```python
from build123d import *

# Parameters (mm, degrees)
EXTRUDE_1_DEPTH     = 6
SKETCH_2_W          = 1
SKETCH_2_H          = 3.5
CUT_EXTRUDE_1_DEPTH = 30.086079144
SKETCH_3_W          = 1
SKETCH_3_H          = 3.5
CUT_EXTRUDE_2_DEPTH = 6


with BuildPart() as part:
    # 草图1 → 凸台-拉伸1 (new body)
    with BuildSketch(Plane(origin=(0, 0, 0), x_dir=(1, 0, 0), z_dir=(0, 1, 0))):
        Polygon((0, 0), (26.5, 0), (26.5, 8.5), (27, 8.5), (27, -0.5), (0, -0.5), align=None)
    extrude(amount=EXTRUDE_1_DEPTH)

    # 草图2 → 切除-拉伸1 (cut, through all)
    with BuildSketch(Plane.XY.offset(0.5)):
        with Locations((1.5, 3)):
            Rectangle(SKETCH_2_W, SKETCH_2_H)
        with Locations((4.5, 3)):
            Rectangle(SKETCH_2_W, SKETCH_2_H)
        with Locations((7.5, 3)):
            Rectangle(SKETCH_2_W, SKETCH_2_H)
        with Locations((10.5, 3)):
            Rectangle(SKETCH_2_W, SKETCH_2_H)
        with Locations((13.5, 3)):
            Rectangle(SKETCH_2_W, SKETCH_2_H)
        with Locations((16.5, 3)):
            Rectangle(SKETCH_2_W, SKETCH_2_H)
        with Locations((19.5, 3)):
            Rectangle(SKETCH_2_W, SKETCH_2_H)
        with Locations((22.5, 3)):
            Rectangle(SKETCH_2_W, SKETCH_2_H)
        with Locations((25.5, 3)):
            Rectangle(SKETCH_2_W, SKETCH_2_H)
    extrude(amount=-CUT_EXTRUDE_1_DEPTH, mode=Mode.SUBTRACT)

    # 草图3 → 切除-拉伸2 (cut)
    with BuildSketch(Plane(origin=(27, 0, 0), x_dir=(0, 0, -1), z_dir=(1, 0, 0))):
        with Locations((1, 3)):
            Rectangle(SKETCH_3_W, SKETCH_3_H)
        with Locations((4, 3)):
            Rectangle(SKETCH_3_W, SKETCH_3_H)
        with Locations((7, 3)):
            Rectangle(SKETCH_3_W, SKETCH_3_H)
    extrude(amount=-CUT_EXTRUDE_2_DEPTH, mode=Mode.SUBTRACT)


solid = part.part
```
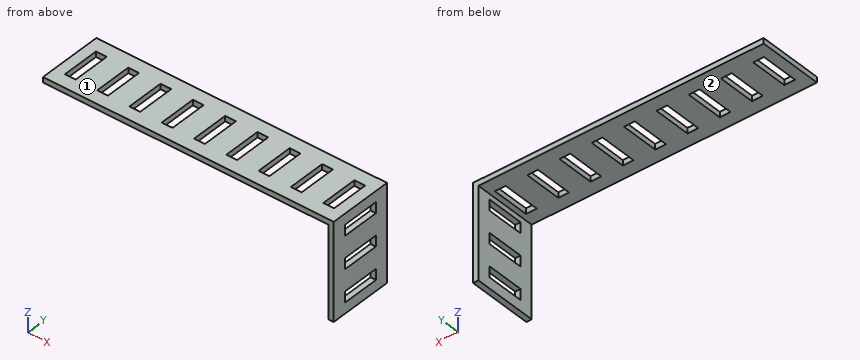
Check sheet for the modelled part. Datum: model origin and axes. Units: mm. Face numbers are marked on the shaded views. A direction names the side the tool comes from. Round coordinates to 2 decimals unless told otherwise and drop trailing zeros. Loops run counter-clockwise (first coordinate to the right, second up) from the corner with the lowest first, then second, coordinate; pieces in that order, holes last. Notation, with made-up numbers: M -15.5,-25 L 33.5,-25 A10 cw 33.5,-19 Z; hole C 41,-3 d4. An arc over 180 degrees is marked long. Answer as a JSON object with one key per item and string values.
1. Scan lines: line 1 (X direction, y = 3.4, z = -5.25); line 2 (Z direction, x = 21, y = 5.7). Record each from-to range of solid material in increasing order.
Reply:
{"line 1": "x = 26.5 to 27", "line 2": "z = 0 to 0.5"}
2. Section check C-C (y = 0.8). Record the boundary of the cut face in (x, z).
Reply:
{"outline": "M 0,0 L 26.5,0 L 26.5,-8.5 L 27,-8.5 L 27,0.5 L 0,0.5 Z"}
3. Section check D-D (z = -8). Record the boundary of the cut face in (x, y), plus the area to 3 significant figures.
Reply:
{"outline": "M 26.5,0 L 27,0 L 27,6 L 26.5,6 Z", "area": "3.00 mm²"}
4. Gauge pin test, flat end, axial feed: P1, Ø1, axis at x = 18, y = 1.5, coming from the -Z side. Record the tip position at first contact, or that the pin passes through.
Reply:
{"P1": "stops at z = 0"}
5. Access from +Z, -Z, +X, -X, +Y, -Y to the whole of each face (thin tool, end or side, straight path). Record for the marked faces 1 and 2.
Reply:
{"face 1": "+Z, +X, -X, +Y, -Y", "face 2": "-Z, -X, +Y, -Y"}
6. Section check B-B (x = 4.75). Record the boundary of the cut face in (y, z).
Reply:
{"outline": "M 0,0 L 1.25,0 L 1.25,0.5 L 0,0.5 Z; M 4.75,0 L 6,0 L 6,0.5 L 4.75,0.5 Z"}
7. Section check A-A (z = -4). Record the boundary of the cut face in (x, y).
Reply:
{"outline": "M 26.5,0 L 27,0 L 27,1.25 L 26.5,1.25 Z; M 26.5,4.75 L 27,4.75 L 27,6 L 26.5,6 Z"}
